from build123d import *

# Parameters (mm, degrees)
CROQUIS1_W              = 110
CROQUIS1_H              = 120
CROQUIS1_R              = 1.5
CROQUIS1_R_2            = 1.75
SALIENTE_EXTRUIR1_DEPTH = 3
CROQUIS4_R              = 1.75
CROQUIS4_R_2            = 1.5
CORTAR_EXTRUIR2_DEPTH   = 10
SALIENTE_EXTRUIR2_DEPTH = 10
CORTAR_EXTRUIR3_DEPTH   = 10
CROQUIS7_R              = 0.875
CROQUIS7_R_2            = 8.25
CORTAR_EXTRUIR5_DEPTH   = 10
REDONDEO4_R             = 3
CORTAR_EXTRUIR6_DEPTH   = 10


with BuildPart() as part:
    # Croquis1 → Saliente-Extruir1 (new body)
    with BuildSketch(Plane.XY):
        with Locations((55, 60)):
            Rectangle(CROQUIS1_W, CROQUIS1_H)
        with Locations((32.5, 82.5)):
            Circle(CROQUIS1_R, mode=Mode.SUBTRACT)
        with Locations(Location((77.5, 82.5, 0), (0, 0, 180))):
            Circle(CROQUIS1_R, mode=Mode.SUBTRACT)
        with Locations((77.5, 37.5)):
            Circle(CROQUIS1_R, mode=Mode.SUBTRACT)
        with Locations(Location((32.5, 37.5, 0), (0, 0, 180))):
            Circle(CROQUIS1_R, mode=Mode.SUBTRACT)
        with Locations((95, 17.5)):
            Circle(CROQUIS1_R_2, mode=Mode.SUBTRACT)
        with Locations((87.5, 25)):
            Circle(CROQUIS1_R_2, mode=Mode.SUBTRACT)
        with Locations(Location((22.5, 25, 0), (0, 0, 180))):
            Circle(CROQUIS1_R_2, mode=Mode.SUBTRACT)
        with Locations(Location((15, 17.5, 0), (0, 0, 180))):
            Circle(CROQUIS1_R_2, mode=Mode.SUBTRACT)
        with Locations(Location((87.5, 95, 0), (0, 0, 180))):
            Circle(CROQUIS1_R_2, mode=Mode.SUBTRACT)
        with Locations(Location((95, 102.5, 0), (0, 0, 180))):
            Circle(CROQUIS1_R_2, mode=Mode.SUBTRACT)
        with Locations((15, 102.5)):
            Circle(CROQUIS1_R_2, mode=Mode.SUBTRACT)
        with Locations((22.5, 95)):
            Circle(CROQUIS1_R_2, mode=Mode.SUBTRACT)
    extrude(amount=SALIENTE_EXTRUIR1_DEPTH)

    # Croquis4 → Cortar-Extruir2 (cut)
    # profile 1 of 4: a face of its own
    with BuildSketch(Plane(origin=(0, 0, 0), x_dir=(-1, 0, 0), z_dir=(0, 0, -1))):
        with Locations((-32.5, 82.5)):
            Circle(CROQUIS4_R)
        with Locations((-32.5, 82.5)):
            Circle(CROQUIS4_R_2, mode=Mode.SUBTRACT)
    # profile 2 of 4: a face of its own
    with BuildSketch(Plane(origin=(0, 0, 0), x_dir=(-1, 0, 0), z_dir=(0, 0, -1))):
        with Locations((-32.5, 37.5)):
            Circle(CROQUIS4_R)
        with Locations((-32.5, 37.5)):
            Circle(CROQUIS4_R_2, mode=Mode.SUBTRACT)
    # profile 3 of 4: a face of its own
    with BuildSketch(Plane(origin=(0, 0, 0), x_dir=(-1, 0, 0), z_dir=(0, 0, -1))):
        with Locations((-77.5, 82.5)):
            Circle(CROQUIS4_R)
        with Locations((-77.5, 82.5)):
            Circle(CROQUIS4_R_2, mode=Mode.SUBTRACT)
    # profile 4 of 4: a face of its own
    with BuildSketch(Plane(origin=(0, 0, 0), x_dir=(-1, 0, 0), z_dir=(0, 0, -1))):
        with Locations((-77.5, 37.5)):
            Circle(CROQUIS4_R)
        with Locations((-77.5, 37.5)):
            Circle(CROQUIS4_R_2, mode=Mode.SUBTRACT)
    extrude(amount=-CORTAR_EXTRUIR2_DEPTH, mode=Mode.SUBTRACT)

    # Croquis5 → Saliente-Extruir2 (add)
    with BuildSketch(Plane(origin=(0, 0, 0), x_dir=(-1, 0, 0), z_dir=(0, 0, -1))):
        with BuildLine():
            Line((-22.5, 78), (-22.5, 77.5))
            ThreePointArc((-22.5, 77.5), (-22.646446609, 77.146446609), (-23, 77))
            Line((-23, 77), (-77, 77))
            ThreePointArc((-77, 77), (-77.353553391, 77.146446609), (-77.5, 77.5))
            Line((-77.5, 77.5), (-77.5, 78))
            ThreePointArc((-77.5, 78), (-77.353553391, 78.353553391), (-77, 78.5))
            Line((-77, 78.5), (-23, 78.5))
            ThreePointArc((-23, 78.5), (-22.646446609, 78.353553391), (-22.5, 78))
        make_face()
        with BuildLine():
            Line((-92.2, 49.5), (-91.3, 49.5))
            ThreePointArc((-91.3, 49.5), (-91.087867966, 49.587867966), (-91, 49.8))
            Line((-91, 49.8), (-91, 70.2))
            ThreePointArc((-91, 70.2), (-91.087867966, 70.412132034), (-91.3, 70.5))
            Line((-91.3, 70.5), (-92.2, 70.5))
            ThreePointArc((-92.2, 70.5), (-92.412132034, 70.412132034), (-92.5, 70.2))
            Line((-92.5, 70.2), (-92.5, 49.8))
            ThreePointArc((-92.5, 49.8), (-92.412132034, 49.587867966), (-92.2, 49.5))
        make_face()
        with BuildLine():
            Line((-17.5, 70.2), (-17.5, 49.8))
            ThreePointArc((-17.5, 49.8), (-17.587867966, 49.587867966), (-17.8, 49.5))
            Line((-17.8, 49.5), (-18.7, 49.5))
            ThreePointArc((-18.7, 49.5), (-18.912132034, 49.587867966), (-19, 49.8))
            Line((-19, 49.8), (-19, 70.2))
            ThreePointArc((-19, 70.2), (-18.912132034, 70.412132034), (-18.7, 70.5))
            Line((-18.7, 70.5), (-17.8, 70.5))
            ThreePointArc((-17.8, 70.5), (-17.587867966, 70.412132034), (-17.5, 70.2))
        make_face()
        with BuildLine():
            Line((-76, 42.7), (-76, 41.8))
            ThreePointArc((-76, 41.8), (-75.912132034, 41.587867966), (-75.7, 41.5))
            Line((-75.7, 41.5), (-24.3, 41.5))
            ThreePointArc((-24.3, 41.5), (-24.087867966, 41.587867966), (-24, 41.8))
            Line((-24, 41.8), (-24, 42.7))
            ThreePointArc((-24, 42.7), (-24.087867966, 42.912132034), (-24.3, 43))
            Line((-24.3, 43), (-75.7, 43))
            ThreePointArc((-75.7, 43), (-75.912132034, 42.912132034), (-76, 42.7))
        make_face()
    extrude(amount=SALIENTE_EXTRUIR2_DEPTH)

    # Croquis6 → Cortar-Extruir3 (cut)
    with BuildSketch(Plane(origin=(0, 0, 0), x_dir=(-1, 0, 0), z_dir=(0, 0, -1))):
        with BuildLine():
            Line((-82, 71), (-28, 71))
            ThreePointArc((-28, 71), (-25.878679656, 70.121320344), (-25, 68))
            Line((-25, 68), (-25, 52))
            ThreePointArc((-25, 52), (-25.878679656, 49.878679656), (-28, 49))
            Line((-28, 49), (-82, 49))
            ThreePointArc((-82, 49), (-84.121320344, 49.878679656), (-85, 52))
            Line((-85, 52), (-85, 68))
            ThreePointArc((-85, 68), (-84.121320344, 70.121320344), (-82, 71))
        make_face()
        with BuildLine():
            Line((-71.709897982, 84.148550743), (-69.876564649, 82.148550743))
            ThreePointArc((-69.876564649, 82.148550743), (-69.207582851, 81.669303614), (-68.402256369, 81.5))
            Line((-68.402256369, 81.5), (-41.597743631, 81.5))
            ThreePointArc((-41.597743631, 81.5), (-40.792417149, 81.669303614), (-40.123435351, 82.148550743))
            Line((-40.123435351, 82.148550743), (-38.290102018, 84.148550743))
            ThreePointArc((-38.290102018, 84.148550743), (-37.933713912, 86.305326482), (-39.764410298, 87.5))
            Line((-39.764410298, 87.5), (-70.235589702, 87.5))
            ThreePointArc((-70.235589702, 87.5), (-72.066286088, 86.305326482), (-71.709897982, 84.148550743))
        make_face()
        with BuildLine():
            Line((-39.764410298, 32.5), (-70.235589702, 32.5))
            ThreePointArc((-70.235589702, 32.5), (-72.066286088, 33.694673518), (-71.709897982, 35.851449257))
            Line((-71.709897982, 35.851449257), (-69.876564649, 37.851449257))
            ThreePointArc((-69.876564649, 37.851449257), (-69.207582851, 38.330696386), (-68.402256369, 38.5))
            Line((-68.402256369, 38.5), (-41.597743631, 38.5))
            ThreePointArc((-41.597743631, 38.5), (-40.792417149, 38.330696386), (-40.123435351, 37.851449257))
            Line((-40.123435351, 37.851449257), (-38.290102018, 35.851449257))
            ThreePointArc((-38.290102018, 35.851449257), (-37.933713912, 33.694673518), (-39.764410298, 32.5))
        make_face()
    extrude(amount=-CORTAR_EXTRUIR3_DEPTH, mode=Mode.SUBTRACT)

    # Croquis7 → Cortar-Extruir5 (cut)
    with BuildSketch(Plane(origin=(0, 0, 0), x_dir=(-1, 0, 0), z_dir=(0, 0, -1))):
        with BuildLine():
            Line((-60.5, 0), (-49.5, 0))
            Line((-49.5, 0), (-49.5, 4.5))
            ThreePointArc((-49.5, 4.5), (-49.792893219, 5.207106781), (-50.5, 5.5))
            Line((-50.5, 5.5), (-59.5, 5.5))
            ThreePointArc((-59.5, 5.5), (-60.207106781, 5.207106781), (-60.5, 4.5))
            Line((-60.5, 4.5), (-60.5, 0))
        make_face()
        with Locations((-76.075, 19.575)):
            Circle(CROQUIS7_R)
        with Locations((-76.075, 1.425)):
            Circle(CROQUIS7_R)
        with Locations((-33.925, 1.425)):
            Circle(CROQUIS7_R)
        with Locations((-33.925, 19.575)):
            Circle(CROQUIS7_R)
        with Locations((-68.3, 10.5)):
            Circle(CROQUIS7_R_2)
        with Locations((-41.7, 10.5)):
            Circle(CROQUIS7_R_2)
    extrude(amount=-CORTAR_EXTRUIR5_DEPTH, mode=Mode.SUBTRACT)

    # Redondeo4
    redondeo4_edges = [part.edges().sort_by_distance(p)[0] for p in [
        (60.5, 0, 1.5),
        (49.5, 0, 1.5),
    ]]
    fillet(redondeo4_edges, radius=REDONDEO4_R)

    # Croquis9 → Cortar-Extruir6 (cut)
    with BuildSketch(Plane(origin=(0, 0, 0), x_dir=(-1, 0, 0), z_dir=(0, 0, -1))):
        with BuildLine():
            Line((-66.350200723, 90.5), (-43.649799277, 90.5))
            ThreePointArc((-43.649799277, 90.5), (-39.623166866, 91.346518071), (-36.278257875, 93.742753715))
            Line((-36.278257875, 93.742753715), (-18.979043258, 112.614624206))
            ThreePointArc((-18.979043258, 112.614624206), (-6.26313434, 113.167489811), (-5.710268735, 100.451580893))
            Line((-5.710268735, 100.451580893), (-9.839056422, 95.94744887))
            ThreePointArc((-9.839056422, 95.94744887), (-11.787263247, 92.815432645), (-12.46751502, 89.190202585))
            Line((-12.46751502, 89.190202585), (-12.46751502, 28.864878962))
            ThreePointArc((-12.46751502, 28.864878962), (-12.127389133, 27.052263932), (-11.153285721, 25.486255819))
            Line((-11.153285721, 25.486255819), (-5.710268735, 19.548419107))
            ThreePointArc((-5.710268735, 19.548419107), (-9.732013396, 6.983331017), (-22.297101486, 11.005075679))
            Line((-22.297101486, 11.005075679), (-23.26284586, 12.058614996))
            ThreePointArc((-23.26284586, 12.058614996), (-24.362523006, 12.31486519), (-25, 11.382890367))
            Line((-25, 11.382890367), (-25, 4))
            ThreePointArc((-25, 4), (-26.171572875, 1.171572875), (-29, 0))
            Line((-29, 0), (0, 0))
            Line((0, 0), (0, 120))
            Line((0, 120), (-110, 120))
            Line((-110, 120), (-110, 0))
            Line((-110, 0), (-81, 0))
            ThreePointArc((-81, 0), (-83.828427125, 1.171572875), (-85, 4))
            Line((-85, 4), (-85, 11.382890367))
            ThreePointArc((-85, 11.382890367), (-85.637476994, 12.31486519), (-86.73715414, 12.058614996))
            Line((-86.73715414, 12.058614996), (-87.702898514, 11.005075679))
            ThreePointArc((-87.702898514, 11.005075679), (-100.267986604, 6.983331017), (-104.289731265, 19.548419107))
            Line((-104.289731265, 19.548419107), (-98.846714279, 25.486255819))
            ThreePointArc((-98.846714279, 25.486255819), (-97.872610867, 27.052263932), (-97.53248498, 28.864878962))
            Line((-97.53248498, 28.864878962), (-97.53248498, 89.190202585))
            ThreePointArc((-97.53248498, 89.190202585), (-98.212736753, 92.815432645), (-100.160943578, 95.94744887))
            Line((-100.160943578, 95.94744887), (-104.289731265, 100.451580893))
            ThreePointArc((-104.289731265, 100.451580893), (-103.73686566, 113.167489811), (-91.020956742, 112.614624206))
            Line((-91.020956742, 112.614624206), (-73.721742125, 93.742753715))
            ThreePointArc((-73.721742125, 93.742753715), (-70.376833134, 91.346518071), (-66.350200723, 90.5))
        make_face()
    extrude(amount=-CORTAR_EXTRUIR6_DEPTH, mode=Mode.SUBTRACT)


solid = part.part
The model under review builds one solid part; all positions refer to its coordinate system, in mm. A direction names the side the tool comes from. Give positions to 0.01 mm unless a question says otherwise; leave off trailing zeros. Loops run counter-clockwise (first coordinate to the right, second up) from the corner with the lowest first, then second, coordinate; pieces in that order, holes last. Notation, with made-up numbers: (-7, 75.5) -> (8, 75.5) arc R9 ccw to (8, 82.5) -> close; hole circle Ø1 at (20, -24.5). An arc over 180 degrees is marked (long way). Answer as a JSON object with one key per item and string values. Group by question number.
Q1. Take a section at B-B (y = 58.5). Write out the cut boundary in (x, z), plus the area to 3 significant figures.
Q2. Tool access review of faces 4 (the flat face through (97.532, 59, 1)), 5 (the cylindrical face through (37.921, 33.724, 1.479)), 6 (the flat face through (91, 60, -5)): name each direction out of +Z, -Z, +X, -X, +Y, -Y from which nothing blocks a thin tool from reaching the whole face with its end or side.
Q3. Take a section at C-C (z = -6.25). State how many separate pieces and enclosed holes the cut face has, plus the area to 3 significant figures.
Q4. Insertion check: pin 1 (2.5 mm diameter, centred on x = 57, z = 1.5, fed in from -Y); pin 2 (1 mm diameter, centred on x = 63, y = 16.5, fed in from -Z); pin 3 (3 mm diameter, centred on x = 95, y = 102.5, fed in from +Z); pin 4 (0.7 mm diameter, centred on y = 42.5, z = -5.5, fed in from +X). Each pin has a flat end and moves straight along its axis. Give the tip position at first contact, or say it passes through.
Q5. Take a section at A-A (x = 57). Write out the cut boundary in (y, z), plus the area to 3 significant figures.
Q6. Wall thickness on line 1 along Y through (x, z) = (65, -4.5); line 2 along Y through (x, z) = (53, 1.75); line 3 along X through (y, z) = (82.5, 2.3): over which ranges is each line inside the solid? List them lowest first.
Q7. Draft analysis for pull direction Y (two halves, no side actions). For faces 1 (the cylindrical face through (23.79, 23.82, 1.48)), 2 (the flat face through (92.5, 60, -5)), 3 (the flat face through (38, 0, 1)), state which applies: pulls with the +Y half, pulls with the -Y half, needs draft (parallel to the pull), parting line crosses it, or undercut.
Q8. Take a section at D-D (y = 102.5). Write out the cut boundary in (x, z).
Answer below:
{
 "1": {"outline": "(12.47, 0) -> (17.5, 0) -> (17.5, -10) -> (19, -10) -> (19, 0) -> (25, 0) -> (25, 3) -> (12.47, 3) -> close; (85, 0) -> (91, 0) -> (91, -10) -> (92.5, -10) -> (92.5, 0) -> (97.53, 0) -> (97.53, 3) -> (85, 3) -> close", "area": "105 mm2"},
 "2": {"face 4": "+Z, -Z, +X", "face 5": "+Z, -Z", "face 6": "-Z, +Y, -Y"},
 "3": {"separate pieces": "4", "enclosed holes": "0", "area": "223 mm2"},
 "4": {"pin 1": "stops at y = 5.5", "pin 2": "stops at z = 0", "pin 3": "passes through", "pin 4": "stops at x = 76"},
 "5": {"outline": "(5.5, 0) -> (32.5, 0) -> (32.5, 3) -> (5.5, 3) -> close; (38.5, 0) -> (41.5, 0) -> (41.5, -10) -> (43, -10) -> (43, 0) -> (49, 0) -> (49, 3) -> (38.5, 3) -> close; (71, 0) -> (77, 0) -> (77, -10) -> (78.5, -10) -> (78.5, 0) -> (81.5, 0) -> (81.5, 3) -> (71, 3) -> close; (87.5, 0) -> (90.5, 0) -> (90.5, 3) -> (87.5, 3) -> close", "area": "183 mm2"},
 "6": {"line 1": "y = 41.5 to 43, 77 to 78.5", "line 2": "y = 5.5 to 32.5, 38.5 to 49, 71 to 81.5, 87.5 to 90.5", "line 3": "x = 12.47 to 30.75, 34.25 to 39.8, 70.2 to 75.75, 79.25 to 97.53"},
 "7": {"face 1": "undercut", "face 2": "needs draft", "face 3": "pulls with the -Y half"},
 "8": {"outline": "(4.3, 0) -> (13.25, 0) -> (13.25, 3) -> (4.3, 3) -> close; (16.75, 0) -> (28.25, 0) -> (28.25, 3) -> (16.75, 3) -> close; (81.75, 0) -> (93.25, 0) -> (93.25, 3) -> (81.75, 3) -> close; (96.75, 0) -> (105.7, 0) -> (105.7, 3) -> (96.75, 3) -> close"}
}
